Here's how the part is built. I have some questions about the finished solid (model axes, mm). A direction names the side the tool comes from. Round coordinates to 2 decimals unless told otherwise and drop trailing zeros. Loops run counter-clockwise (first coordinate to the right, second up) from the corner with the lowest first, then second, coordinate; pieces in that order, holes last. Notation, with made-up numbers: (80, -20) - (93, -20) arc R21 cw to (93, 11) - close; hole circle Ø2 at (-31.75, 6.25). An arc over 180 degrees is marked (long way). Answer as a JSON object with one key per item and string values. Group by question number.
1) Which directions (+Z, -Z, +X, -X, +Y, -Y) give clear straight access to the entire face, cutting with the end or side of a thin tool? Please do faces 3 (the face through (-31.562, 19.466, 44.83)), 4 (the face through (-65, -22, 47.7)).
2) I want a section at A-A, the plane z = 44.9. Please give me the cut outline in (x, y) (3 decimals).
3) If we mould it in two halves opening along X, with no side actions, what happens to faces 1 (the face through (-58.477, 19.474, 44.831)), 2 (the face through (-23, 9, 42.7))? For each: pulls with the +X half, pulls with the -X half, needs draft (parallel to the pull), parting line crosses it, or undercut.
4) Will these pins go through, and if not, where does the flat tip stop? P1, Ø12, axis at x = -43.5, y = -13.5, coming from the +Z side; P2, Ø2, axis at x = -56, y = 22.5, coming from the +Z side; P3, Ø3, axis at y = -23, z = 45, coming from the +X side; P4, Ø1.5, axis at y = 5, z = 45.5, coming from the +X side.
5) If I drill on line 1 along X through (y, z) = (0.5, 43.2); line 2 along Y through (x, z) = (-34.5, 44.25); line 3 along Y through (x, z) = (-32, 46.5), over which ranges is the centre line in solid material (lowest first)? Write a range as [from, to].
from build123d import *

# Parameters (mm, degrees)
PAD013_DEPTH       = 5
CHAMFER004_SIZE2   = 9
CHAMFER004_SIZE    = 1.5
POCKET005_DEPTH    = 5
SKETCH029_R        = 1.6
POCKET006_DEPTH    = 5
POLARPATTERN_COUNT = 4


with BuildPart() as part:
    # Sketch027 → Pad013 (new body)
    with BuildSketch(Plane.XY):
        with BuildLine():
            ThreePointArc((0, 29.9), (-21.142493, 21.142493), (-29.9, 0))
            Line((-29.9, 0), (-20.5, 0))
            ThreePointArc((0, 20.5), (-14.495689, 14.495689), (-20.5, 0))
            Line((0, 29.9), (0, 20.5))
        make_face()
    extrude(amount=PAD013_DEPTH)

    # Chamfer004
    chamfer004_edges = [part.edges().sort_by_distance(p)[0] for p in [
        (-14.495689, 14.495689, 5),
    ]]
    chamfer004_side = part.faces().sort_by_distance((-14.495689, 14.495689, 2.5))[0]
    chamfer(chamfer004_edges, length=CHAMFER004_SIZE, length2=CHAMFER004_SIZE2, reference=chamfer004_side)

    # Sketch015 (on Face6 of Pad013) → Pocket005 (cut)
    with BuildSketch(Plane.XY.offset(5)):
        with BuildLine():
            ThreePointArc((0, 20.5), (-14.495689, 14.495689), (-20.5, 0))
            Line((-20.5, 0), (-23.25, 0))
            ThreePointArc((-19.791981, 12.2), (-22.368796, 6.340306), (-23.25, 0))
            ThreePointArc((-19.791981, 12.2), (-19.466026, 13.456827), (-19.866411, 14.691959))
            ThreePointArc((-14.691475, 19.881138), (-19.458765, 19.460387), (-19.866411, 14.691959))
            ThreePointArc((-14.691475, 19.881138), (-13.458731, 19.47346), (-12.2, 19.791981))
            ThreePointArc((0, 23.25), (-6.340306, 22.368796), (-12.2, 19.791981))
            Line((0, 20.5), (0, 23.25))
        make_face()
    extrude(amount=-POCKET005_DEPTH, mode=Mode.SUBTRACT)

    # Sketch029 (on Face3 of Pocket005) → Pocket006 (cut)
    with BuildSketch(Plane(origin=(-16.776703, 16.775598, 4.528711), x_dir=(-0.705669, 0.705678, 0.063645), z_dir=(0.045003, -0.045005, 0.997973))):
        with Locations((-16.95, 16.95)):
            Circle(SKETCH029_R)
    extrude(amount=-POCKET006_DEPTH, mode=Mode.SUBTRACT)

    # PolarPattern: part ×4 about axis
    polarpattern_axis = Axis((0, 0, 0), (0, 0, 1))


with BuildPart() as part_1:
    add(part.part)
    for i in range(1, POLARPATTERN_COUNT):
        add(part.part.rotate(polarpattern_axis, i * 360 / POLARPATTERN_COUNT))


with BuildPart() as part_2:
    # Body003 placement: moved
    add(part_1.part.moved(Location((-45, 0, 42.7))))


solid = part_2.part
Outcome:
{
 "1": {"face 3": "+Z, -Z", "face 4": "+Z, +X, -X, +Y, -Y"},
 "2": {"outline": "(-74.9, 0) arc R29.9 ccw to (-45, -29.9) arc R29.9 ccw to (-15.1, 0) arc R29.9 ccw to (-45, 29.9) arc R29.9 ccw to start; hole (-68.25, 0) arc R23.25 ccw to (-64.792, -12.2) arc R2.32 cw to (-64.881, -14.691) arc R3.72 ccw to (-59.692, -19.866) arc R2.32 cw to (-57.2, -19.792) arc R23.25 ccw to (-45, -23.25) arc R23.25 ccw to (-32.8, -19.792) arc R2.32 cw to (-30.309, -19.881) arc R3.72 ccw to (-25.134, -14.692) arc R2.32 cw to (-25.208, -12.2) arc R23.25 ccw to (-21.75, 0) arc R23.25 ccw to (-25.208, 12.2) arc R2.32 cw to (-25.119, 14.691) arc R3.72 ccw to (-30.308, 19.866) arc R2.32 cw to (-32.8, 19.792) arc R23.25 ccw to (-45, 23.25) arc R23.25 ccw to (-57.2, 19.792) arc R2.32 cw to (-59.691, 19.881) arc R3.72 ccw to (-64.866, 14.692) arc R2.32 cw to (-64.792, 12.2) arc R23.25 ccw to start"},
 "3": {"face 1": "undercut", "face 2": "needs draft"},
 "4": {"P1": "through", "P2": "z = 47.12", "P3": "x = -24.22", "P4": "x = -15.4"},
 "5": {"line 1": "[-74.9, -68.24], [-21.76, -15.1]", "line 2": "[-28, -20.74], [20.74, 28]", "line 3": "[-26.93, -19.5], [19.5, 26.93]"}
}
